Here's how the part is built. I have some questions about the finished solid (model axes, mm). A direction names the side the tool comes from. Round coordinates to 2 decimals unless told otherwise and drop trailing zeros. Write each loop counter-clockwise with the first axis right and the second up, starting at its lowest first coordinate (ties: lowest second). Pieces come first, ordered by that corner, then holes. Notation, with made-up numbers: (-11, 33.5) -> (0, 33.5) arc R16 cw to (0, 42.5) -> close; hole circle Ø11 at (-11.5, 75.25). An arc over 180 degrees is marked (long way). Answer in a Markdown table with one row per item. Add a question column.
Autodesk Inventor part; units mm, degrees
ref_plane "YZ Plane" through (0, 0, 0) normal (1, 0, 0) x (0, 1, 0)
ref_plane "XZ Plane" through (0, 0, 0) normal (0, 1, 0) x (-1, 0, 0)
ref_plane "XY Plane" through (0, 0, 0) normal (0, 0, 1) x (1, 0, 0)
sketch "Sketch2" plane through (0, 0, 0) normal (1, 0, 0) x (0, 1, 0)
  line L0 (-6.35, 6.35) -> (6.35, 6.35)
  line L1 (6.35, 6.35) -> (6.35, -6.35)
  line L2 (6.35, -6.35) -> (-6.35, -6.35)
  line L3 (-6.35, -6.35) -> (-6.35, 6.35)
  line L4 (-6.35, 6.35) -> (6.35, -6.35) construction
  line L5 (6.35, 6.35) -> (-6.35, -6.35) construction
  line L6 (-4.7625, 4.7625) -> (4.7625, 4.7625)
  line L7 (4.7625, 4.7625) -> (4.7625, -4.7625)
  line L8 (4.7625, -4.7625) -> (-4.7625, -4.7625)
  line L9 (-4.7625, -4.7625) -> (-4.7625, 4.7625)
  line L10 (-4.7625, 4.7625) -> (4.7625, -4.7625) construction
  line L11 (4.7625, 4.7625) -> (-4.7625, -4.7625) construction
  line L12 (4.7625, 4.7625) -> (6.35, 4.7625)
  line L13 (4.7625, -4.7625) -> (6.35, -4.7625)
  point P0 (0, 0)
  dimension "d0" = 12.7
  dimension "d1" = 12.7
  dimension "d2" = 9.525
  dimension "d3" = 9.525
extrude "Extrusion1" add sketch "Sketch2" along normal mid plane 14.2875 contours L0 L1 L12 L6 L9 L8 L13 L2 L3
sketch "Sketch3" plane through (-7.1437, -4.7625, 4.7625) normal (0, 1, 0) x (1, 0, 0)
  line L0 (0, 0) -> (14.2875, 0)
  line L1 (14.2875, 9.525) -> (14.2875, 0)
  line L2 (0, 9.525) -> (14.2875, 9.525)
  line L3 (0, 0) -> (0, 9.525)
  line L4 (-2.8575, 4.7625) -> (17.145, 4.7625)
  line L5 (7.1437, 13.6525) -> (7.1437, -4.1275)
  circle A0 centre (2.6988, 4.7625) radius 1.5875
  point P0 (7.1437, 4.7625)
  dimension "d6" = 3.175
  dimension "d7" = 4.445
extrude "Extrusion2" cut sketch "Sketch3" against normal through all contours A0 L4 | L4 A0
mirror "Mirror1" about plane through (0, 0, 0) normal (1, 0, 0) of "Extrusion2"
properties part number "halfinchCChannel"
Item 1: If we section it at A-A on y = 2.5: Please give me the cut outline in (x, z), then the cut area to 3 significant figures.
Item 2: If we section it at C-C on x = -3.25: Please give me the cut outline in (y, z), then the cut area to 3 significant figures.
Item 3: On a 3-axis mill with a long thin cutter (end or side, diameter ignored), from which of +Z, -Z, +X, -X, +Y, -Y can I reach the whole of each face in a straight line? I mean faces 1 (the flat face through (0, 1, 4.762)), 2 (the flat face through (7.144, -5, 0)). Say none if no direction works.
Item 4: I need wall thicknesses on line 1 along Z through (x, y) = (5.75, -2); line 2 along Z through (x, y) = (-4.5, -5.25); line 3 along Y through (x, z) = (-1.5, -1.75). Which ranges of each line are inside material? Lowest first, please. Write a range as from..to.
Item 5: For P1, Ø5, axis at x = -4.44, z = 0, coming from the +Y side, with a flat end and sliding along its axis, tell me the tip position at first contact or that it passes through.
Item 6: If we mould it in two halves opening along Z, with no side actions, what happens to faces 3 (the flat face through (0, 0, 6.35)), 4 (the flat face through (0, 0, -6.35)), 5 (the flat face through (0, -4.762, 0))? For each: pulls with the +Z half, pulls with the -Z half, needs draft (parallel to the pull), parting line crosses it, or undercut.
Item 7: If we section it at D-D on x = 4: Please give me the cut outline in (y, z).
Item 8: If we section it at B-B on z = 0: Please give me the cut outline in (x, y), then the cut area to 3 significant figures.
Results list:
| question | item | result |
|---|---|---|
| 1 | outline | (-7.14, -6.35) -> (7.14, -6.35) -> (7.14, -4.76) -> (-7.14, -4.76) -> close; (-7.14, 4.76) -> (7.14, 4.76) -> (7.14, 6.35) -> (-7.14, 6.35) -> close |
| 1 | area | 45.4 mm² |
| 2 | outline | (-6.35, -6.35) -> (6.35, -6.35) -> (6.35, -4.76) -> (-4.76, -4.76) -> (-4.76, -1.05) -> (-6.35, -1.05) -> close; (-6.35, 1.05) -> (-4.76, 1.05) -> (-4.76, 4.76) -> (6.35, 4.76) -> (6.35, 6.35) -> (-6.35, 6.35) -> close |
| 2 | area | 52.1 mm² |
| 3 | face 1 | +X, -X, +Y |
| 3 | face 2 | +Z, -Z, +X, +Y, -Y |
| 4 | line 1 | -6.35..-4.76, 4.76..6.35 |
| 4 | line 2 | -6.35..-1.59, 1.59..6.35 |
| 4 | line 3 | -6.35..-4.76 |
| 5 | P1 | y = -4.76 |
| 6 | face 3 | pulls with the +Z half |
| 6 | face 4 | pulls with the -Z half |
| 6 | face 5 | undercut |
| 7 | outline | (-6.35, -6.35) -> (6.35, -6.35) -> (6.35, -4.76) -> (-4.76, -4.76) -> (-4.76, -1.52) -> (-6.35, -1.52) -> close; (-6.35, 1.52) -> (-4.76, 1.52) -> (-4.76, 4.76) -> (6.35, 4.76) -> (6.35, 6.35) -> (-6.35, 6.35) -> close |
| 8 | outline | (-7.14, -6.35) -> (-6.03, -6.35) -> (-6.03, -4.76) -> (-7.14, -4.76) -> close; (-2.86, -6.35) -> (2.86, -6.35) -> (2.86, -4.76) -> (-2.86, -4.76) -> close; (6.03, -6.35) -> (7.14, -6.35) -> (7.14, -4.76) -> (6.03, -4.76) -> close |
| 8 | area | 12.6 mm² |
